```python
from build123d import *

# Parameters (mm, degrees)
SKETCH_1_R          = 17.5
SKETCH_1_R_2        = 1.75
EXTRUDE_1_DEPTH     = 4
CUT_EXTRUDE_1_DEPTH = 3
SKETCH_3_R          = 9
EXTRUDE_2_DEPTH     = 7
CUT_EXTRUDE_2_DEPTH = 2
SKETCH_6_R          = 4
EXTRUDE_3_DEPTH     = 3
CHAMFER_1_SIZE      = 1
CHAMFER_2_SIZE      = 0.5


with BuildPart() as part:
    # Эскиз1 → Бобышка-Вытянуть1 (new body)
    with BuildSketch(Plane(origin=(0, 0, 0), x_dir=(1, 0, 0), z_dir=(0, 1, 0))):
        Circle(SKETCH_1_R)
        with Locations((13, 0)):
            Circle(SKETCH_1_R_2, mode=Mode.SUBTRACT)
        with Locations((0, -13)):
            Circle(SKETCH_1_R_2, mode=Mode.SUBTRACT)
        with Locations((-13, 0)):
            Circle(SKETCH_1_R_2, mode=Mode.SUBTRACT)
        with Locations((0, 13)):
            Circle(SKETCH_1_R_2, mode=Mode.SUBTRACT)
    extrude(amount=EXTRUDE_1_DEPTH)

    # Эскиз2 → Вырез-Вытянуть1 (cut)
    with BuildSketch(Plane(origin=(0, 4, 0), x_dir=(1, 0, 0), z_dir=(0, 1, 0))):
        Polygon((3.348631561, 13), (1.674315781, 15.9), (-1.674315781, 15.9), (-3.348631561, 13), (-1.674315781, 10.1), (1.674315781, 10.1), align=None)
        Polygon((-13, -3.348631561), (-10.1, -1.674315781), (-10.1, 1.674315781), (-13, 3.348631561), (-15.9, 1.674315781), (-15.9, -1.674315781), align=None)
        Polygon((15.9, -1.674315781), (13, -3.348631561), (10.1, -1.674315781), (10.1, 1.674315781), (13, 3.348631561), (15.9, 1.674315781), align=None)
        Polygon((1.674315781, -10.1), (3.348631561, -13), (1.674315781, -15.9), (-1.674315781, -15.9), (-3.348631561, -13), (-1.674315781, -10.1), align=None)
    extrude(amount=-CUT_EXTRUDE_1_DEPTH, mode=Mode.SUBTRACT)

    # Эскиз3 → Бобышка-Вытянуть2 (add)
    with BuildSketch(Plane(origin=(0, 4, 0), x_dir=(1, 0, 0), z_dir=(0, 1, 0))):
        Circle(SKETCH_3_R)
        with BuildLine():
            Line((-1.852025918, -2.1), (1.852025918, -2.1))
            ThreePointArc((1.852025918, -2.1), (0, 2.8), (-1.852025918, -2.1))
        make_face(mode=Mode.SUBTRACT)
    extrude(amount=EXTRUDE_2_DEPTH)

    # Эскиз4 → Вырез-Вытянуть2 (cut)
    with BuildSketch(Plane(origin=(0, 4, 0), x_dir=(1, 0, 0), z_dir=(0, 1, 0))):
        with BuildLine():
            Line((-1.852025918, -2.1), (1.852025918, -2.1))
            ThreePointArc((1.852025918, -2.1), (0, 2.8), (-1.852025918, -2.1))
        make_face()
    extrude(amount=-CUT_EXTRUDE_2_DEPTH, mode=Mode.SUBTRACT)

    # Эскиз6 → Бобышка-Вытянуть3 (add)
    with BuildSketch(Plane(origin=(0, 11, 0), x_dir=(1, 0, 0), z_dir=(0, 1, 0))):
        Circle(SKETCH_6_R)
        with BuildLine():
            Line((-1.852025918, -2.1), (1.852025918, -2.1))
            ThreePointArc((1.852025918, -2.1), (0, 2.8), (-1.852025918, -2.1))
        make_face(mode=Mode.SUBTRACT)
    extrude(amount=EXTRUDE_3_DEPTH)

    # Фаска1
    chamfer_1_edges = [part.edges().sort_by_distance(p)[0] for p in [
        (-9, 11, 0),
    ]]
    chamfer(chamfer_1_edges, length=CHAMFER_1_SIZE)

    # Фаска2
    chamfer_2_edges = [part.edges().sort_by_distance(p)[0] for p in [
        (0, 14, -2.8),
        (0, 14, 2.1),
    ]]
    chamfer(chamfer_2_edges, length=CHAMFER_2_SIZE)


solid = part.part
```
For this review, take the finished solid that the model builds, in its own axes (mm). A direction names the side the tool comes from. Round coordinates to 2 decimals unless told otherwise and drop trailing zeros. Order: outer loops, then holes, each group sorted by start corner. A loop starts at its lowest first (then second) coordinate and runs counter-clockwise, first axis right, second up.
Q1. We need section C-C, the plane x = 0. State how many separate pieces and enclosed holes the cut face has, plus the area to 3 significant figures.
Findings below:
separate pieces: 3
enclosed holes: 0
area: 188 mm2
Q2. Mouldability with a two-part tool opening along Z and no side actions: class faces 1 (the flat face through (8, 4, 8)), 2 (the conical face through (0.102, 13.635, -2.934)), 3 (the cylindrical face through (-0.867, 12.479, 3.905)) as pulls with the +Z half, pulls with the -Z half, needs draft (parallel to the pull), parting line crosses it, or undercut.
Findings below:
face 1: needs draft
face 2: undercut
face 3: parting line crosses it
Q3. Wall thickness on line 1 (Z direction, x = 0, y = 0.6); line 2 (Z direction, x = 0, y = 6); line 3 (X direction, y = 0.4, z = -13): over which ranges is each line inside the solid? List them lowest first.
Findings below:
line 1: z = -17.5 to -14.75, -11.25 to 11.25, 14.75 to 17.5
line 2: z = -9 to -2.8, 2.1 to 9
line 3: x = -11.72 to -1.75, 1.75 to 11.72
Q4. Machinability: for faces 4 (the flat face through (0, 3, 10.1)), 5 (the cylindrical face through (-13.887, 1.972, 10.648)), which of the approach directions +Z, -Z, +X, -X, +Y, -Y give a long, thin tool a straight path to every point of the face, cutting with its end or side? Answer none if there is none.
Findings below:
face 4: +Y
face 5: +Y, -Y
Q5. Insertion check: P1, Ø1.5, axis at x = 3.5, y = 4.5, coming from the -Z side; P2, Ø7.5, axis at x = 0, z = 0, coming from the +Y side; P3, Ø5, axis at y = 10.5, z = -8.5, coming from the -X side; P4, Ø1.5, axis at y = 12, z = 3.5, coming from the +X side. Each pin has a flat end and moves straight along its axis. Give the tip position at first contact, or say it passes through.
Findings below:
P1: stops at z = -17.25
P2: stops at y = 14
P3: stops at x = -6.66
P4: stops at x = 2.9
Q6. We need section A-A, the plane x = -12. Give the boundary of the cut face in (y, z), plus the area to 3 significant figures.
Findings below:
outline: (0, -12.74) - (4, -12.74) - (4, -2.77) - (1, -2.77) - (1, -1.44) - (0, -1.44) - close; (0, 1.44) - (1, 1.44) - (1, 2.77) - (4, 2.77) - (4, 12.74) - (0, 12.74) - close
area: 82.4 mm2
Q7. We need section B-B, the plane y = 9.5. Give the boundary of the cut face in (x, z).
Findings below:
outline: circle Ø18 at (0, 0); hole (-1.85, 2.1) arc R2.8 ccw (long way) to (1.85, 2.1) - close
